Check sheet for the modelled part. Datum: model origin and axes. Units: mm. A direction names the side the tool comes from. Round coordinates to 2 decimals unless told otherwise and drop trailing zeros. Write each loop counter-clockwise with the first axis right and the second up, starting at its lowest first coordinate (ties: lowest second). Pieces come first, ordered by that corner, then holes. Notation, with made-up numbers: M 10.5,21.25 L 38.5,21.25 A7 cw 38.5,25.25 Z; hole C 42,60.25 d9. An arc over 180 degrees is marked long. Answer in a Markdown table with one row per item.
```python
from build123d import *

# Parameters (mm, degrees)
SKETCH1_R          = 3
EXTRUDE1_DEPTH     = 12
SKETCH6_R          = 5
EXTRUDE2_DEPTH     = 6
CUT_EXTRUDE1_DEPTH = 3.75
CHAMFER1_SIZE      = 0.5


with BuildPart() as part:
    # Sketch1 → Extrude1 (new body)
    with BuildSketch(Plane.XY):
        Circle(SKETCH1_R)
    extrude(amount=-EXTRUDE1_DEPTH)

    # Sketch4 → Cut-Revolve1 (revolve, cut)
    with BuildSketch(Plane(origin=(0, 0, 0), x_dir=(0, 0, -1), z_dir=(1, 0, 0)), mode=Mode.PRIVATE) as cut_revolve1_sk:
        Polygon((0.632650852, 3), (0, 2.096480947), (0, 3), align=None)
    revolve(cut_revolve1_sk.sketch.rotate(Axis((0, 0, 0), (0, 0, -1)), 90), axis=Axis((0, 0, 0), (0, 0, -1)), mode=Mode.SUBTRACT)

    # Sketch6 → Extrude2 (add)
    with BuildSketch(Plane(origin=(0, 0, -12), x_dir=(-1, 0, 0), z_dir=(0, 0, -1))):
        Circle(SKETCH6_R)
    extrude(amount=EXTRUDE2_DEPTH)

    # Sketch7 → Cut-Extrude1 (cut)
    with BuildSketch(Plane(origin=(0, 0, -18), x_dir=(-1, 0, 0), z_dir=(0, 0, -1))):
        Polygon((0, 2.886751346), (-2.5, 1.443375673), (-2.5, -1.443375673), (0, -2.886751346), (2.5, -1.443375673), (2.5, 1.443375673), align=None)
    extrude(amount=-CUT_EXTRUDE1_DEPTH, mode=Mode.SUBTRACT)

    # Chamfer1
    chamfer1_edges = [part.edges().sort_by_distance(p)[0] for p in [
        (5, 0, -12),
        (5, 0, -18),
    ]]
    chamfer(chamfer1_edges, length=CHAMFER1_SIZE)


solid = part.part
```
1. Scan lines: L1, parallel to Z at x = -3.25, y = -1.25; L2, parallel to Y at x = 1, z = -14.75; L3, parallel to Y at x = 2, z = -15.5. Record each from-to range of solid material in increasing order.
Found:
| item | result |
|---|---|
| L1 | z = -18 to -12 |
| L2 | y = -4.9 to -2.31, 2.31 to 4.9 |
| L3 | y = -4.58 to -1.73, 1.73 to 4.58 |
2. Section check A-A, the plane y = 0. Record the cut outline in (x, z), and give its area (3 significant figures).
Found:
| item | result |
|---|---|
| outline | M -5,-17.5 L -4.5,-18 L -2.5,-18 L -2.5,-14.25 L 2.5,-14.25 L 2.5,-18 L 4.5,-18 L 5,-17.5 L 5,-12.5 L 4.5,-12 L 3,-12 L 3,-0.63 L 2.1,0 L -2.1,0 L -3,-0.63 L -3,-12 L -4.5,-12 L -5,-12.5 Z |
| area | 112 mm2 |
3. Section check B-B, the plane z = -8.75. Record the cut outline in (x, y).
Found:
| item | result |
|---|---|
| outline | C 0,0 d6 |
4. Access from +Z, -Z, +X, -X, +Y, -Y to the whole of each face (thin tool, end or side, straight path). Record for faces 1 (the face through (-1.267, 2.155, -16.151)), 2 (the face through (-2, -2, -18)), 3 (the face through (-1, -3, -12)).
Found:
| item | result |
|---|---|
| face 1 | -Z |
| face 2 | -Z, +X, -X, +Y, -Y |
| face 3 | +Z |
5. Go/stop test with flat-tipped pins: pin 1 (5 mm diameter, centred on x = -3.5, z = -6, fed in from +Y); pin 2 (4 mm diameter, centred on y = -2.5, z = -8.5, fed in from +X); pin 3 (3 mm diameter, centred on x = 1, y = -3.5, fed in from +Z). Record where each tip stops, or that it passes through.
Found:
| item | result |
|---|---|
| pin 1 | stops at y = 2.83 |
| pin 2 | stops at x = 2.96 |
| pin 3 | stops at z = -0.03 |
